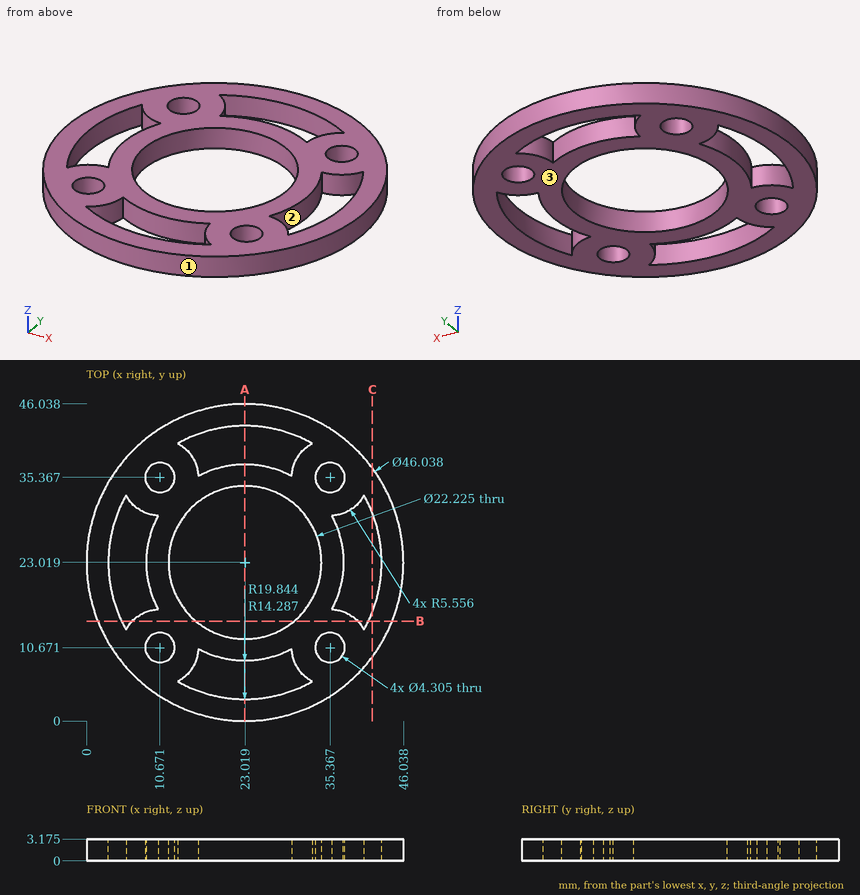
Answer from the drawing. Dimensions are ordinates in mm from the lowest x, y and z of the part. Coordinates: 2 decimals unless noted, no trailing zeros. Loops run counter-clockwise (first coordinate to the right, second up) from the corner with the lowest first, then second, coordinate; pieces in that order, holes last.
1) For a pull along Y with two mould halves and no side action, classify the marked faces 1, 2 and 3 as +Y half, -Y half, draft (parallel to the pull), parting line (faces both ways), or undercut.
Results:
face 1: parting line
face 2: undercut
face 3: draft
2) Flat-ended cylindrical pins translate along their axes: pin 1 (1 mm diameter, centred on y = 8.5, z = 0.5, fed in from -X); pin 2 (1 mm diameter, centred on y = 10.5, z = 2.5, fed in from -X). Find the tip coordinate at first contact, or state that the pin passes through.
Results:
pin 1: stops at x = 4.76
pin 2: stops at x = 3.39
3) Section A-A (x = 23) is taken. Give the vertices of the cut face in (y, z) (1 decimal).
Results:
outline: (0, 0) - (3.2, 0) - (3.2, 3.2) - (0, 3.2) - close; (8.7, 0) - (11.9, 0) - (11.9, 3.2) - (8.7, 3.2) - close; (34.1, 0) - (37.3, 0) - (37.3, 3.2) - (34.1, 3.2) - close; (42.9, 0) - (46, 0) - (46, 3.2) - (42.9, 3.2) - close
4) Section C-C (x = 41.5) is taken. Give the vertices of the cut face in (y, z) (1 decimal).
Results:
outline: (9.3, 0) - (15.8, 0) - (15.8, 3.2) - (9.3, 3.2) - close; (30.2, 0) - (36.7, 0) - (36.7, 3.2) - (30.2, 3.2) - close
5) Consider probe 1 along Y at (x, z) = (22.5, 0.2) (1 decimal); probe 2 along X at (y, z) = (35.5, 2.7) (1 decimal). Determine where each line is inside the solid, lowest interval first.
Results:
probe 1: y = 0 to 3.2, 8.7 to 11.9, 34.1 to 37.3, 42.9 to 46
probe 2: x = 3.7 to 8.5, 12.8 to 33.2, 37.5 to 42.4
6) Section B-B (y = 14.5) is taken. Give the vertices of the cut face in (x, z) (1 decimal).
Results:
outline: (1.6, 0) - (5.1, 0) - (5.1, 3.2) - (1.6, 3.2) - close; (6.6, 0) - (15.9, 0) - (15.9, 3.2) - (6.6, 3.2) - close; (30.2, 0) - (39.4, 0) - (39.4, 3.2) - (30.2, 3.2) - close; (40.9, 0) - (44.4, 0) - (44.4, 3.2) - (40.9, 3.2) - close
